from build123d import *

# Parameters (mm, degrees)
SKETCH_1_R          = 2
EXTRUDE_1_DEPTH     = 20
SKETCH_2_R          = 1
CUT_EXTRUDE_1_DEPTH = 11
CHAMFER_1_SIZE      = 0.1


with BuildPart() as part:
    # 草图1 → 凸台-拉伸1 (new body)
    with BuildSketch(Plane.XY):
        Circle(SKETCH_1_R)
    extrude(amount=EXTRUDE_1_DEPTH)

    # 草图2 → 切除-拉伸1 (cut)
    with BuildSketch(Plane(origin=(0, 0, 0), x_dir=(-1, 0, 0), z_dir=(0, 0, -1))):
        Circle(SKETCH_2_R)
    extrude(amount=-CUT_EXTRUDE_1_DEPTH, mode=Mode.SUBTRACT)

    # 倒角1
    chamfer_1_edges = [part.edges().sort_by_distance(p)[0] for p in [
        (-2, 0, 0),
        (-2, 0, 20),
    ]]
    chamfer(chamfer_1_edges, length=CHAMFER_1_SIZE)


solid = part.part
Read the model definition and answer for the solid it produces. Units are mm, in the model's axes. Coordinates: 2 decimals unless noted, no trailing zeros. Write each loop counter-clockwise with the first axis right and the second up, starting at its lowest first coordinate (ties: lowest second). Pieces come first, ordered by that corner, then holes. Notation, with made-up numbers: M 2.5,-25 L 12.5,-25 A36 cw 12.5,13 Z; hole C 14.25,31.25 d7. An arc over 180 degrees is marked long. Use a Markdown table: item, result.
Q1. Determine the mould class of faces 1 (the face through (0, 0, 11)), 2 (the face through (1, -1, 0)), 3 (the face through (0, -2, 10)), 4 (the face through (0, -1, 5)) for opening direction Y: released by +Y, released by -Y, zero draft, split by the parting line, or undercut.
Answer block:
| item | result |
|---|---|
| face 1 | undercut |
| face 2 | zero draft |
| face 3 | split by the parting line |
| face 4 | undercut |
Q2. The part is cut by section C-C, the plane z = 9.5. Write down the section's boundary in (x, y), then the cut area to 3 significant figures.
Answer block:
| item | result |
|---|---|
| outline | C 0,0 d4; hole C 0,0 d2 |
| area | 9.42 mm2 |
Q3. Straight lines are drawn through the part: L1, parallel to Y at x = 0, z = 7.75; L2, parallel to Z at x = 0.65, y = 0; L3, parallel to X at y = -0.8, z = 9. For each, find the intervals that lie inside material, in ascending order. Write a range as [from, to].
Answer block:
| item | result |
|---|---|
| L1 | y = [-2, -1], [1, 2] |
| L2 | z = [11, 20] |
| L3 | x = [-1.83, -0.6], [0.6, 1.83] |
Q4. The part is cut by section A-A, the plane y = 0. Write down the section's boundary in (x, z), then the cut area to 3 significant figures.
Answer block:
| item | result |
|---|---|
| outline | M -2,0.1 L -1.9,0 L -1,0 L -1,11 L 1,11 L 1,0 L 1.9,0 L 2,0.1 L 2,19.9 L 1.9,20 L -1.9,20 L -2,19.9 Z |
| area | 58.0 mm2 |
Q5. Each of these flat-tipped pins is pushed along its axis until it touches: pin 1 Ø1.5 at (x, z) = (1, 7) entering from +Y; pin 2 Ø1 at (x, z) = (-1, 4.5) entering from -Y. Where does it stop, or does it pass through?
Answer block:
| item | result |
|---|---|
| pin 1 | stops at y = 1.98 |
| pin 2 | stops at y = -1.94 |
